Source: CAD feature listing. Evaluate the final solid. Frame: model axes, mm. Face numbers are marked on the shaded views. A direction names the side the tool comes from. Coordinates: 2 decimals unless noted, no trailing zeros. Write each loop counter-clockwise with the first axis right and the second up, starting at its lowest first coordinate (ties: lowest second). Pieces come first, ordered by that corner, then holes. Notation, with made-up numbers: M -24.5,85.5 L 10.5,85.5 A18 ccw 10.5,116.5 Z; hole C -38.75,-15.75 d6. An arc over 180 degrees is marked long. One line per item, written item: value. Start each with the question number.
Item 1: Ray query, L1, parallel to X at y = 17.9, z = -6; L2, parallel to Y at x = 13.5, z = -7.5; L3, parallel to Y at x = 18, z = -8. Return the intervals inside material, ascending. Write a range as from..to.
Item 2: Pin query (flat end, axial travel): P1, Ø5, axis at y = 13, z = -3.5, coming from the +X side; P2, Ø1.8, axis at x = 3, z = -9, coming from the +Y side; P3, Ø1.5, axis at x = 11.5, y = 24, coming from the +Z side. Return the tip coordinate at first contact, or that it passes through.
Item 3: Cut plane D-D, the plane y = 29.5. Output: boundary loops of the cut face in (x, z), then the cut area to 3 significant figures.
Item 4: Cut plane A-A, the plane y = 18.5. Output: boundary loops of the cut face in (x, z).
Item 5: Set-up query: the marked faces 1, 2, 3, 4 and 5. Return all of +Z, -Z, +X, -X, +Y, -Y with unobstructed straight access to the full face (end or side cutting, diameter ignored); none if empty.
Item 6: Cut plane B-B, the plane x = 19. Output: boundary loops of the cut face in (y, z), then the cut area to 3 significant figures.
Item 7: Cut plane C-C, the plane z = -2.5. Output: boundary loops of the cut face in (x, y), then the cut area to 3 significant figures.
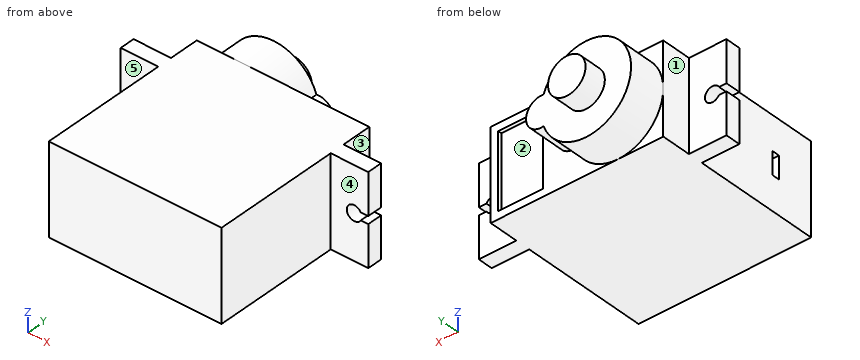
```python
from build123d import *

# Parameters (mm, degrees)
SKETCH1_W           = 23
SKETCH1_H           = 12
BOSS_EXTRUDE1_DEPTH = 23
BOSS_EXTRUDE2_DEPTH = 5
SKETCH3_W           = 12
SKETCH3_H           = 2
BOSS_EXTRUDE3_DEPTH = 5
CUT_EXTRUDE1_START  = -5
CUT_EXTRUDE1_DEPTH  = 41.902646142
SKETCH5_R           = 2.5
BOSS_EXTRUDE4_DEPTH = 3
SKETCH6_W           = 6
SKETCH6_H           = 10
CUT_EXTRUDE2_DEPTH  = 0.5
SKETCH7_W           = 3
SKETCH7_H           = 1
CUT_EXTRUDE3_DEPTH  = 1


with BuildPart() as part:
    # Sketch1 → Boss-Extrude1 (new body)
    with BuildSketch(Plane(origin=(0, 0, 0), x_dir=(1, 0, 0), z_dir=(0, 1, 0))):
        with Locations((11.5, 6)):
            Rectangle(SKETCH1_W, SKETCH1_H)
    extrude(amount=BOSS_EXTRUDE1_DEPTH)

    # Sketch2 → Boss-Extrude2 (add)
    with BuildSketch(Plane(origin=(0, 23, 0), x_dir=(1, 0, 0), z_dir=(0, 1, 0))):
        with BuildLine():
            ThreePointArc((11.666666667, 7.972026594), (0, 6), (11.666666667, 4.027973406))
            ThreePointArc((11.666666667, 4.027973406), (14, 6), (11.666666667, 7.972026594))
        make_face()
    extrude(amount=BOSS_EXTRUDE2_DEPTH)

    # Sketch3 → Boss-Extrude3 (add)
    with BuildSketch(Plane(origin=(23, 0, 0), x_dir=(0, 0, -1), z_dir=(1, 0, 0))):
        with Locations((6, 18)):
            Rectangle(SKETCH3_W, SKETCH3_H)
    boss_extrude3 = extrude(amount=BOSS_EXTRUDE3_DEPTH)

    # Sketch4 → Cut-Extrude1 (cut)
    with BuildSketch(Plane(origin=(0, 19, 0), x_dir=(1, 0, 0), z_dir=(0, 1, 0)).offset(CUT_EXTRUDE1_START)):
        with BuildLine():
            Line((28, 6.5), (27, 6.5))
            ThreePointArc((27, 6.5), (25.133974596, 6), (27, 5.5))
            Line((27, 5.5), (28, 5.5))
            Line((28, 5.5), (28, 6.5))
        make_face()
    cut_extrude1 = extrude(amount=CUT_EXTRUDE1_DEPTH, mode=Mode.SUBTRACT)

    # Mirror3: Boss-Extrude3, Cut-Extrude1 across plane
    add(boss_extrude3.mirror(Plane.ZY.offset(-11.5)))
    add(cut_extrude1.mirror(Plane.ZY.offset(-11.5)), mode=Mode.SUBTRACT)

    # Sketch5 → Boss-Extrude4 (add)
    with BuildSketch(Plane(origin=(0, 28, 0), x_dir=(1, 0, 0), z_dir=(0, 1, 0))):
        with Locations(Location((6, 6, 0), (0, 0, 270))):
            Circle(SKETCH5_R)
    extrude(amount=BOSS_EXTRUDE4_DEPTH)

    # Sketch6 → Cut-Extrude2 (cut)
    with BuildSketch(Plane(origin=(0, 23, 0), x_dir=(1, 0, 0), z_dir=(0, 1, 0))):
        with Locations((19, 6)):
            Rectangle(SKETCH6_W, SKETCH6_H)
    extrude(amount=-CUT_EXTRUDE2_DEPTH, mode=Mode.SUBTRACT)

    # Sketch7 → Cut-Extrude3 (cut)
    with BuildSketch(Plane.ZY):
        with Locations((-6, 5.5)):
            Rectangle(SKETCH7_W, SKETCH7_H)
    extrude(amount=-CUT_EXTRUDE3_DEPTH, mode=Mode.SUBTRACT)


solid = part.part
```
From the geometry:
1. L1: x = -2.13..25.13
1. L2: y = 0..23
1. L3: y = 0..22.5
2. P1: stops at x = 23
2. P2: stops at y = 28
2. P3: stops at z = -2.33
3. outline: C 6,-6 d5
3. area: 19.6 mm²
4. outline: M -5,-12 L 28,-12 L 28,-6.5 L 27,-6.5 A1 cw long 27,-5.5 L 28,-5.5 L 28,0 L -5,0 L -5,-5.5 L -4,-5.5 A1 cw long -4,-6.5 L -5,-6.5 Z
5. face 1: +Z, -Z, -X, +Y
5. face 2: +Y
5. face 3: +Z, -Z, +X, +Y
5. face 4: +Z, -Z, +X, -Y
5. face 5: +Z, -Z, -X, -Y
6. outline: M 0,-12 L 23,-12 L 23,-11 L 22.5,-11 L 22.5,-1 L 23,-1 L 23,0 L 0,0 Z
6. area: 271 mm²
7. outline: M -5,17 L 0,17 L 0,0 L 23,0 L 23,17 L 28,17 L 28,19 L 23,19 L 23,23 L 22,23 L 22,22.5 L 16,22.5 L 16,23 L 10.87,23 L 10.87,28 L 1.13,28 L 1.13,23 L 0,23 L 0,19 L -5,19 Z
7. area: 595 mm²
